The drawing under review shows one solid part. Ordinate dimensions are in mm from its lowest x, y, z. Coordinates: 2 decimals unless noted, no trailing zeros. Write each loop counter-clockwise with the first axis right and the second up, starting at its lowest first coordinate (ties: lowest second). Pieces come first, ordered by that corner, then holes.
1) Add section D-D, the plane y = 203. State the section outline as (x, z) points.
2) Add section B-B, the plane z = 6.5. State the section outline as (x, y) points.
3) Add section C-C, the plane x = 190. State the section outline as (y, z) points, then the cut area to 3 significant figures.
4) Add section A-A, the plane y = 328.54. State the section outline as (x, z) points, then the cut area to 3 significant figures.
5) For line 1 (Y direction, x = 69.5, z = 10.25); line 2 (X direction, y = 377, z = 3.5); line 3 (X direction, y = 410, z = 7), list the stretches that pass through material, from the lowest coordinate up.
6) For P1, Ø2, axis at y = 265.5, z = 11, coming from the +X side; P2, Ø1, axis at y = 348.5, z = 7.5, coming from the +X side; P3, Ø2, axis at x = 209, y = 110, coming from the -Z side, all flat-tipped, find the tip position at first contact; note any pin that passes through.
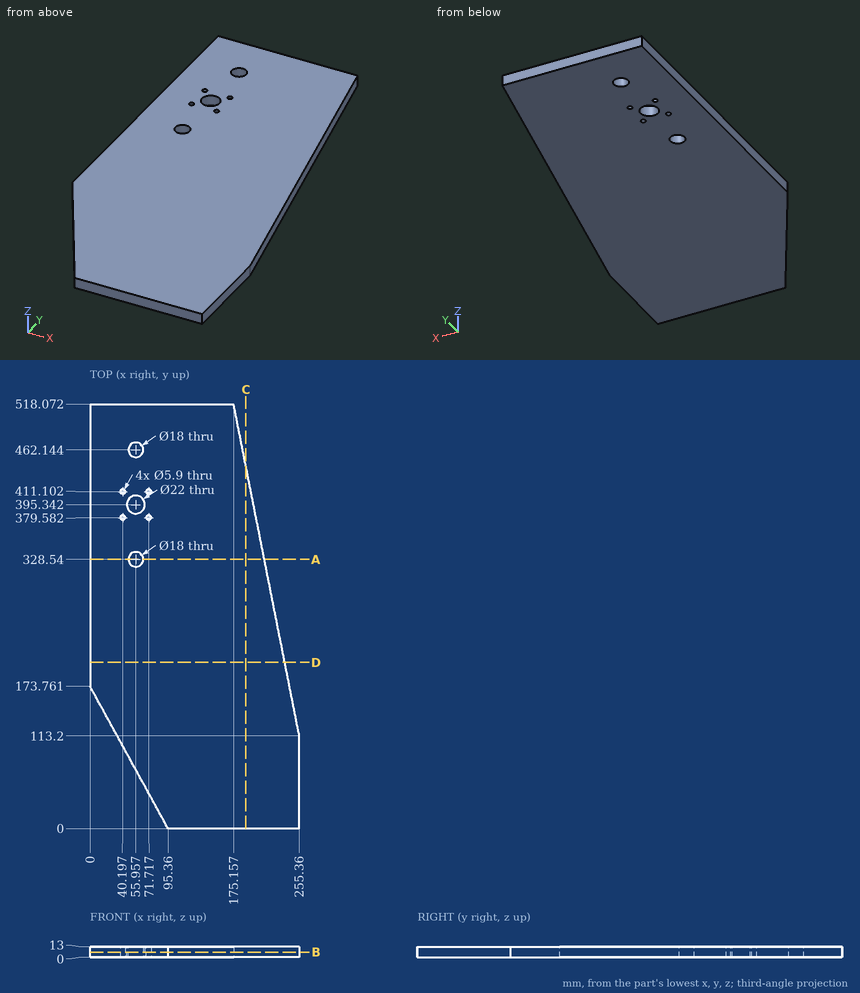
Geometry results:
1. outline: (0, 0) - (237.57, 0) - (237.57, 13) - (0, 13) - close
2. outline: (0, 173.76) - (95.36, 0) - (255.36, 0) - (255.36, 113.2) - (175.16, 518.07) - (0, 518.07) - close; hole circle Ø5.9 at (40.2, 379.58); hole circle Ø5.9 at (40.2, 411.1); hole circle Ø22 at (55.96, 395.34); hole circle Ø18 at (55.96, 328.54); hole circle Ø18 at (55.96, 462.14); hole circle Ø5.9 at (71.72, 379.58); hole circle Ø5.9 at (71.72, 411.1)
3. outline: (0, 0) - (443.14, 0) - (443.14, 13) - (0, 13) - close
3. area: 5,760 mm2
4. outline: (0, 0) - (46.96, 0) - (46.96, 13) - (0, 13) - close; (64.96, 0) - (212.7, 0) - (212.7, 13) - (64.96, 13) - close
4. area: 2,530 mm2
5. line 1: y = 47.12 to 377.64, 381.53 to 409.16, 413.05 to 518.07
5. line 2: x = 0 to 38.77, 41.62 to 70.29, 73.14 to 203.1
5. line 3: x = 0 to 37.46, 42.93 to 68.98, 74.45 to 196.57
6. P1: stops at x = 225.39
6. P2: stops at x = 208.85
6. P3: stops at z = 0
